Source: CAD feature listing. Evaluate the final solid. Frame: model axes, mm. Coordinates: 2 decimals unless noted, no trailing zeros. Loops run counter-clockwise (first coordinate to the right, second up) from the corner with the lowest first, then second, coordinate; pieces in that order, holes last.
Item 1: Pull-direction query (X, two-part tool) for faces 1 (the flat face through (3, 1, 2.54)), 2 (the flat face through (12.7, -1, 1)), 3 (the cylindrical face through (8.03, 52.83, 1.25)), 4 (the cylindrical face through (8.03, 39.37, 1.25)); classes: +X half, -X half, draft (parallel to the pull), parting line (faces both ways), or undercut.
Item 2: Section query A-A, the plane z = 0.65. State how many separate pieces and enclosed holes the cut face has, then the cut area to 3 significant figures.
Item 3: Pin query (flat end, axial travel): pin 1 Ø1 at (x, z) = (-1, 2.5) entering from -Y; pin 2 Ø4.5 at (x, y) = (-6.73, 50.8) entering from +Z; pin 3 Ø1.5 at (x, z) = (7, 0.5) entering from +Y; pin 4 Ø1.5 at (x, z) = (3.5, 1.5) entering from +Y. Return the tip coordinate at first contact, or that it passes through.
Item 4: Section query B-B, the plane x = 10.25. Return the cut outline in (y, z).
Item 5: Line query: probe 1 along Y at (x, z) = (-8.25, 0.25); probe 2 along Y at (x, z) = (5, 1.1); probe 3 along Y at (x, z) = (1.25, 1.7) (3 decimals). Output: solid intervals per line, ascending.
```python
from build123d import *

# Parameters (mm, degrees)
F0_R     = 2.413
F1_DEPTH = 2.54
F2_R     = 1.397
F3_DEPTH = 2.541


with BuildPart() as f1:
    # F0 (on Top) → F1 (new body)
    with BuildSketch(Plane.XY):
        with BuildLine():
            Line((12.7, -50.8), (12.7, 50.8))
            ThreePointArc((12.7, 50.8), (0, 63.5), (-12.7, 50.8))
            Line((-12.7, 50.8), (-12.7, -50.8))
            ThreePointArc((-12.7, -50.8), (0, -63.5), (12.7, -50.8))
        make_face()
        with BuildLine():
            Line((4.318, -50.7966617284), (-4.318, -50.7966617284))
            ThreePointArc((-4.318, -50.7966617284), (-8.437248663, -52.5029103914), (-6.731, -48.3836617284))
            Line((-6.731, -48.3836617284), (-6.731, -39.7476617284))
            ThreePointArc((-6.731, -39.7476617284), (-8.437248663, -35.6284130654), (-4.318, -37.3346617284))
            Line((-4.318, -37.3346617284), (4.318, -37.3346617284))
            ThreePointArc((4.318, -37.3346617284), (6.731, -34.9216617284), (9.144, -37.3346617284))
            ThreePointArc((9.144, -37.3346617284), (8.437248663, -39.0409103914), (6.731, -39.7476617284))
            Line((6.731, -39.7476617284), (6.731, -48.3836617284))
            ThreePointArc((6.731, -48.3836617284), (8.437248663, -49.0904130654), (9.144, -50.7966617284))
            ThreePointArc((9.144, -50.7966617284), (6.731, -53.2096617284), (4.318, -50.7966617284))
        make_face(mode=Mode.SUBTRACT)
        with Locations((-6.731, 37.3346617284)):
            Circle(F0_R, mode=Mode.SUBTRACT)
        with Locations((-6.731, 50.7966617284)):
            Circle(F0_R, mode=Mode.SUBTRACT)
        with Locations((6.731, 37.3346617284)):
            Circle(F0_R, mode=Mode.SUBTRACT)
        with Locations((6.731, 50.7966617284)):
            Circle(F0_R, mode=Mode.SUBTRACT)
        with BuildLine():
            ThreePointArc((-6.731, -48.3836617284), (-5.024751337, -49.0904130654), (-4.318, -50.7966617284))
            Line((-4.318, -50.7966617284), (4.318, -50.7966617284))
            ThreePointArc((4.318, -50.7966617284), (5.024751337, -49.0904130654), (6.731, -48.3836617284))
            Line((6.731, -48.3836617284), (6.731, -39.7476617284))
            ThreePointArc((6.731, -39.7476617284), (5.024751337, -39.0409103914), (4.318, -37.3346617284))
            Line((4.318, -37.3346617284), (-4.318, -37.3346617284))
            ThreePointArc((-4.318, -37.3346617284), (-5.024751337, -39.0409103914), (-6.731, -39.7476617284))
            Line((-6.731, -39.7476617284), (-6.731, -48.3836617284))
        make_face()
    extrude(amount=F1_DEPTH)

    # F2 (on face) → F3 (cut, through all)
    with BuildSketch(Plane.XY.offset(2.54)):
        with BuildLine():
            ThreePointArc((0, -1.397), (0.9878281733, -0.9878281733), (1.397, 0))
            ThreePointArc((1.397, 0), (0.9878281733, 0.9878281733), (0, 1.397))
            Line((0, 1.397), (0, -1.397))
        make_face()
        with BuildLine():
            ThreePointArc((1.397, -12.7112130487), (0.9878281733, -11.7233848754), (0, -11.3142130487))
            ThreePointArc((0, -11.3142130487), (-0.9878281733, -13.699041222), (1.397, -12.7112130487))
        make_face()
        with BuildLine():
            ThreePointArc((1.397, 12.6887869513), (-0.9878281733, 13.6766151246), (0, 11.2917869513))
            ThreePointArc((0, 11.2917869513), (0.9878281733, 11.700958778), (1.397, 12.6887869513))
        make_face()
        with BuildLine():
            Line((0, -1.397), (0, 1.397))
            ThreePointArc((0, 1.397), (-1.397, 0), (0, -1.397))
        make_face()
        with BuildLine():
            ThreePointArc((0.9878281733, 45.0534899017), (0, 45.4626617284), (-0.9878281733, 45.0534899017))
            Line((-0.9878281733, 45.0534899017), (0, 44.0656617284))
            Line((0, 44.0656617284), (0.9878281733, 45.0534899017))
        make_face()
        with BuildLine():
            Line((0, 44.0656617284), (-0.9878281733, 45.0534899017))
            ThreePointArc((-0.9878281733, 45.0534899017), (-1.397, 44.0656617284), (-0.9878281733, 43.0778335551))
            Line((-0.9878281733, 43.0778335551), (0, 44.0656617284))
        make_face()
        with BuildLine():
            Line((0.9878281733, 45.0534899017), (0, 44.0656617284))
            Line((0, 44.0656617284), (0.9878281733, 43.0778335551))
            ThreePointArc((0.9878281733, 43.0778335551), (1.2906597069, 43.5310529734), (1.397, 44.0656617284))
            ThreePointArc((1.397, 44.0656617284), (1.2906597069, 44.6002704834), (0.9878281733, 45.0534899017))
        make_face()
        with BuildLine():
            Line((0.9878281733, 43.0778335551), (0, 44.0656617284))
            Line((0, 44.0656617284), (-0.9878281733, 43.0778335551))
            ThreePointArc((-0.9878281733, 43.0778335551), (0, 42.6686617284), (0.9878281733, 43.0778335551))
        make_face()
        with Locations((0, -44.0656617284)):
            Circle(F2_R)
    extrude(amount=-F3_DEPTH, mode=Mode.SUBTRACT)


solid = f1.part
```
Verdict:
1. face 1: draft
1. face 2: +X half
1. face 3: undercut
1. face 4: undercut
2. separate pieces: 1
2. enclosed holes: 13
2. area: 2,910 mm2
3. pin 1: stops at y = -63.49
3. pin 2: passes through
3. pin 3: stops at y = 61.86
3. pin 4: stops at y = 63.2
4. outline: (-58.3, 0) - (58.3, 0) - (58.3, 2.54) - (-58.3, 2.54) - close
5. probe 1: y = -60.46 to -52.67, -48.92 to -39.21, -35.46 to 35.46, 39.21 to 48.92, 52.67 to 60.46
5. probe 2: y = -62.47 to -52.48, -49.12 to -39.02, -35.65 to 35.65, 39.02 to 49.12, 52.48 to 62.47
5. probe 3: y = -63.438 to -44.689, -43.442 to -13.335, -12.087 to -0.624, 0.624 to 12.065, 13.313 to 43.442, 44.689 to 63.438
